from build123d import *

# Parameters (mm, degrees)
BOSS_EXTRUDE1_DEPTH = 1.5
FILLET1_R           = 1


with BuildPart() as part:
    # Sketch1 → Boss-Extrude1 (new body)
    with BuildSketch(Plane(origin=(0, 0, 0), x_dir=(1, 0, 0), z_dir=(0, 1, 0))):
        with BuildLine():
            Line((-22, 10), (22, 10))
            ThreePointArc((22, 10), (24.121320344, 9.121320344), (25, 7))
            Line((25, 7), (25, -7))
            ThreePointArc((25, -7), (24.121320344, -9.121320344), (22, -10))
            Line((22, -10), (-22, -10))
            ThreePointArc((-22, -10), (-24.121320344, -9.121320344), (-25, -7))
            Line((-25, -7), (-25, 7))
            ThreePointArc((-25, 7), (-24.121320344, 9.121320344), (-22, 10))
        make_face()
        with BuildLine():
            Line((-5, 3), (5, 3))
            ThreePointArc((5, 3), (5.707106781, 2.707106781), (6, 2))
            Line((6, 2), (6, -2))
            ThreePointArc((6, -2), (5.707106781, -2.707106781), (5, -3))
            Line((5, -3), (-5, -3))
            ThreePointArc((-5, -3), (-5.707106781, -2.707106781), (-6, -2))
            Line((-6, -2), (-6, 2))
            ThreePointArc((-6, 2), (-5.707106781, 2.707106781), (-5, 3))
        make_face(mode=Mode.SUBTRACT)
    extrude(amount=BOSS_EXTRUDE1_DEPTH)

    # Fillet1
    fillet1_edges = [part.edges().sort_by_distance(p)[0] for p in [
        (5.707106781, 1.5, -2.707106781),
        (0, 1.5, -3),
        (-5.707106781, 1.5, -2.707106781),
        (-6, 1.5, 0),
        (-5.707106781, 1.5, 2.707106781),
        (0, 1.5, 3),
        (5.707106781, 1.5, 2.707106781),
        (6, 1.5, 0),
    ]]
    fillet(fillet1_edges, radius=FILLET1_R)


solid = part.part
Here's how the part is built. I have some questions about the finished solid (model axes, mm). A direction names the side the tool comes from. Round coordinates to 2 decimals unless told otherwise and drop trailing zeros. Loops run counter-clockwise (first coordinate to the right, second up) from the corner with the lowest first, then second, coordinate; pieces in that order, holes last. Notation, with made-up numbers: (-18, 30.25) - (21, 30.25) arc R25 cw to (21, 45.25) - close; hole circle Ø1 at (12, 78). An arc over 180 degrees is marked (long way). One line per question, with ' | ' between items. Start each with the question number.
Q1. I want a section at C-C (y = 1.15). Write out the boundary of the cut face in (x, z).
Q2. For faces 4 (the cylindrical face through (24.1, 0.74, -9.14)), 5 (the cylindrical face through (6.285, 1.199, 0.028)), 6 (the cylindrical face through (-5.699, 0.247, 2.715)), which set-ups out of +Z, -Z, +X, -X, +Y, -Y let a thin tool reach every point of the face, with its end or its side?
Q3. We'd pull the mould along X, two halves only. Please class faces 1 (the flat face through (0, 0, -5)), 2 (the flat face through (25, 1, 0)), 3 (the cylindrical face through (-5.715, 0.247, -2.699)): +X half, -X half, draft (parallel to the pull), parting line (faces both ways), or undercut.
Q4. I want a section at A-A (z = -0.25). Write out the boundary of the cut face in (x, y), then the cut area to 3 significant figures.
Q5. I want a section at B-B (x = -1). Write out the boundary of the cut face in (y, z).
Q6. Please list where these lines run through material, in increasing order: line 1 (X direction, y = 0.75, z = -0.5); line 2 (X direction, y = 1.3, z = 1.5); line 3 (Z direction, x = -6, y = 1.15). Write a range as [from, to].
Response values:
1) outline: (-25, -7) arc R3 ccw to (-22, -10) - (22, -10) arc R3 ccw to (25, -7) - (25, 7) arc R3 ccw to (22, 10) - (-22, 10) arc R3 ccw to (-25, 7) - close; hole (-6.24, -2) arc R1.24 ccw to (-5, -3.24) - (5, -3.24) arc R1.24 ccw to (6.24, -2) - (6.24, 2) arc R1.24 ccw to (5, 3.24) - (-5, 3.24) arc R1.24 ccw to (-6.24, 2) - close
2) face 4: -Z, +X, +Y, -Y | face 5: +Y | face 6: +Y, -Y
3) face 1: draft | face 2: +X half | face 3: undercut
4) outline: (-25, 0) - (-6, 0) - (-6, 0.5) arc R1 ccw to (-7, 1.5) - (-25, 1.5) - close; (6, 0) - (25, 0) - (25, 1.5) - (7, 1.5) arc R1 ccw to (6, 0.5) - close | area: 56.6 mm²
5) outline: (0, -10) - (1.5, -10) - (1.5, -4) arc R1 ccw to (0.5, -3) - (0, -3) - close; (0, 3) - (0.5, 3) arc R1 ccw to (1.5, 4) - (1.5, 10) - (0, 10) - close
6) line 1: x = [-25, -6.03], [6.03, 25] | line 2: x = [-25, -6.4], [6.4, 25] | line 3: z = [-10, -2.73], [2.73, 10]
